Input: dimensioned drawing with shaded views. Units: mm. Origin: part minimum x, y, z. A direction names the side the tool comes from. Give positions to 0.01 mm unless a question says otherwise; leave off trailing zeros. Write each loop counter-clockwise with the first axis right and the second up, starting at its lowest first coordinate (ties: lowest second). Pieces come first, ordered by that corner, then holes.
Q1. Line query: line 1 (Z direction, x = 62.5, y = 73) (1 decimal); line 2 (Y direction, x = 20.5, z = 99) (1 decimal); line 3 (X direction, y = 90, z = 95.5). Output: solid intervals per line, ascending.
Q2. Section A-A (x = 114.3). Return the cut outline in (y, z) (1 decimal), plus the area to 3 significant figures.
Q3. Section D-D (x = 30). Return the cut outline in (y, z) (1 decimal).
Q4. Pin query (flat end, axial travel): pin 1 Ø1 at (y, z) = (39.5, 92.5) entering from +X; pin 2 Ø7.5 at (x, y) = (52.5, 111.5) entering from -Z; pin 3 Ø5 at (x, y) = (176, 20.5) entering from -Z. Return the tip coordinate at first contact, or that it passes through.
Q5. Section C-C (y = 51.5). Return the cut outline in (x, z) (1 decimal).
Q6. Section B-B (z = 34). Return the cut outline in (x, y) (1 decimal).
Q7. Reachability of the marked faces 1 and 2 from +Z, -Z, +X, -X, +Y, -Y: full face, straight path, thin tool, end or side. Return the list, or none.
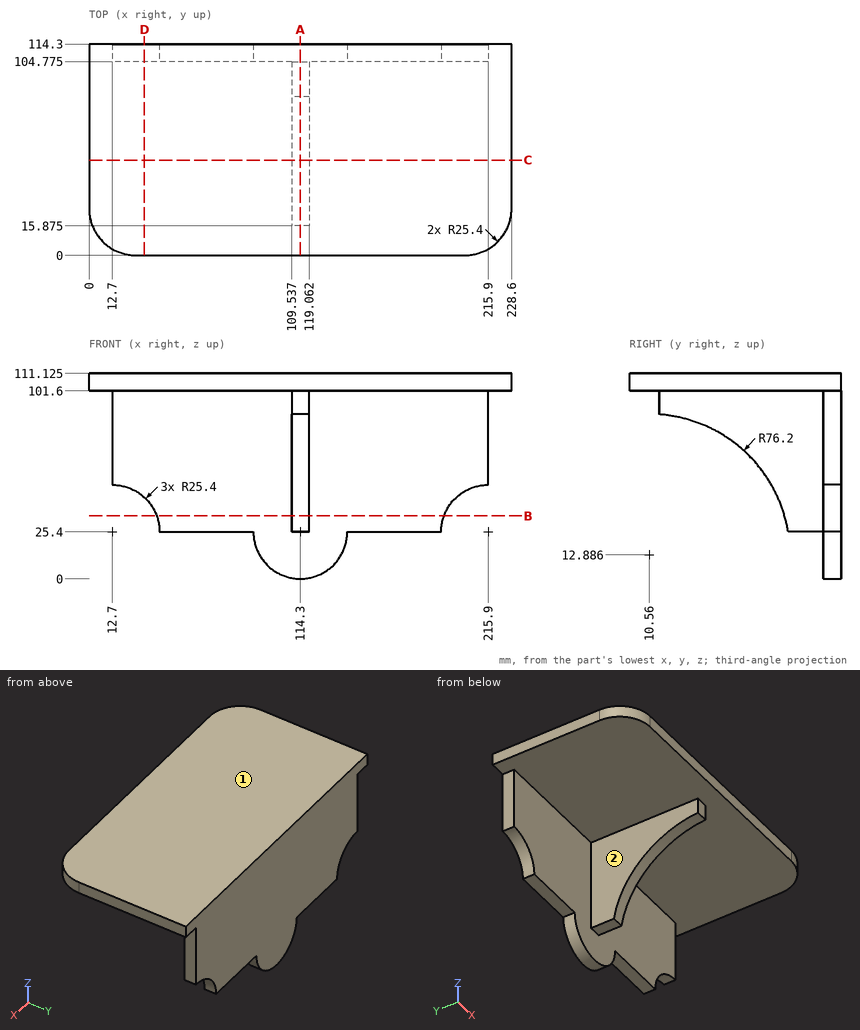
Computed:
1. line 1: z = 101.6 to 111.1
1. line 2: y = 104.8 to 114.3
1. line 3: x = 109.54 to 119.06
2. outline: (0, 101.6) - (15.9, 101.6) - (15.9, 88.9) arc R76.2 cw to (85.7, 25.4) - (104.8, 25.4) - (104.8, 0) - (114.3, 0) - (114.3, 111.1) - (0, 111.1) - close
2. area: 5,560 mm2
3. outline: (0, 101.6) - (104.8, 101.6) - (104.8, 44) - (114.3, 44) - (114.3, 111.1) - (0, 111.1) - close
4. pin 1: stops at x = 119.06
4. pin 2: stops at z = 25.4
4. pin 3: stops at z = 101.6
5. outline: (0, 101.6) - (109.5, 101.6) - (109.5, 77.2) - (119.1, 77.2) - (119.1, 101.6) - (228.6, 101.6) - (228.6, 111.1) - (0, 111.1) - close
6. outline: (36.6, 104.8) - (109.5, 104.8) - (109.5, 83.8) - (119.1, 83.8) - (119.1, 104.8) - (192, 104.8) - (192, 114.3) - (36.6, 114.3) - close
7. face 1: +Z, +X, -X, +Y, -Y
7. face 2: -Z, -X, -Y
